Design review of the part built by this model. Coordinates are the model's own, in mm. Coordinates: 2 decimals unless noted, no trailing zeros. Write each loop counter-clockwise with the first axis right and the second up, starting at its lowest first coordinate (ties: lowest second). Pieces come first, ordered by that corner, then holes. Notation, with made-up numbers: (41.25, 32) -> (92.25, 32) arc R11 ccw to (92.25, 43) -> close; hole circle Ø6 at (-16.5, 19). An arc over 180 degrees is marked (long way). Answer in a Markdown table with one row per item. Add a question column.
Item 1: Take a section at A-A, the plane z = 59.5. Write out the cut boundary in (x, y) (3 decimals).
Item 2: Take a section at C-C, the plane x = 2.55. Give the number of separate pieces and of enclosed holes in the cut face, and give its area (3 significant figures).
Item 3: To check wall thickness, follow line 1 (Y direction, x = 2.7, z = -76); line 2 (Y direction, x = 1.95, z = 0); line 3 (Y direction, x = 0.8, z = 137.5). State the ranges of each line that lie inside material, in increasing order.
Item 4: Take a section at B-B, the plane y = 7.5. Write out the cut boundary in (x, z) (3 decimals), and give its area (3 significant figures).
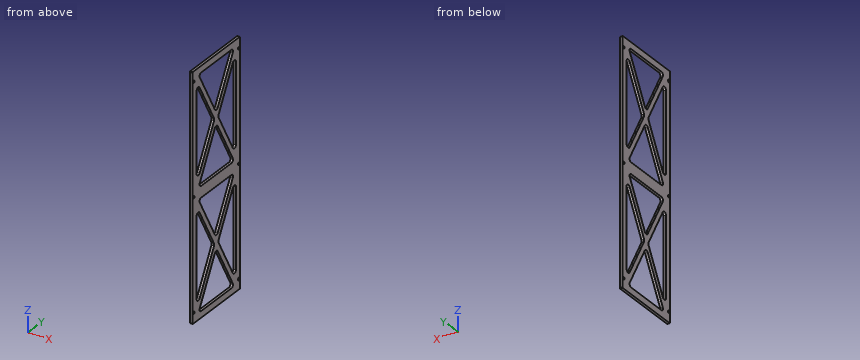
from build123d import *

# Parameters (mm, degrees)
SKETCH2_W            = 300
SKETCH2_H            = 90
BOSS_EXTRUDE1_DEPTH  = 3.175
CUT_EXTRUDE2_DEPTH   = 157.636779286
M3_CLEARANCE_HOLE1_D = 3.2
FILLET1_R            = 3
FILLET2_R            = 1


with BuildPart() as part:
    # Sketch2 → Boss-Extrude1 (new body)
    with BuildSketch(Plane(origin=(0, 0, 0), x_dir=(0, 0, -1), z_dir=(1, 0, 0))):
        Rectangle(SKETCH2_W, SKETCH2_H)
    extrude(amount=BOSS_EXTRUDE1_DEPTH)

    # Sketch4 → Cut-Extrude2 (cut, through all)
    with BuildSketch(Plane(origin=(3.175, 0, 0), x_dir=(0, 0, -1), z_dir=(1, 0, 0))):
        Polygon((-135.758731446, 37), (-13.241268554, 37), (-74.5, 3.4211398), align=None)
        Polygon((-7, 33.5788602), (-7, -33.5788602), (-68.258731446, 0), align=None)
        Polygon((-13.241268554, -37), (-135.758731446, -37), (-74.5, -3.4211398), align=None)
        Polygon((-142, -33.5788602), (-142, 33.5788602), (-80.741268554, 0), align=None)
        Polygon((135.758731446, 37), (13.241268554, 37), (74.5, 3.4211398), align=None)
        Polygon((142, 33.5788602), (80.741268554, 0), (142, -33.5788602), align=None)
        Polygon((135.758731446, -37), (74.5, -3.4211398), (13.241268554, -37), align=None)
        Polygon((7, -33.5788602), (68.258731446, 0), (7, 33.5788602), align=None)
    extrude(amount=-CUT_EXTRUDE2_DEPTH, mode=Mode.SUBTRACT)

    # M3 Clearance Hole1 (through all)
    with Locations(Plane(origin=(3.175, 0, 0), x_dir=(0, 0, -1), z_dir=(1, 0, 0))):
        with Locations((-137.5, 42.61875), (137.5, 42.61875), (137.5, -42.61875), (-137.5, -42.61875), (0, 42.61875), (0, -42.61875)):
            Hole(M3_CLEARANCE_HOLE1_D / 2)

    # Fillet1
    fillet1_edges = [part.edges().sort_by_distance(p)[0] for p in [
        (1.5875, 37, -135.758731446),
        (1.5875, 3.4211398, -74.5),
        (1.5875, 37, -13.241268554),
        (1.5875, 0, 80.741268554),
        (1.5875, -33.5788602, 142),
        (1.5875, 33.5788602, 142),
        (1.5875, 0, 68.258731446),
        (1.5875, 33.5788602, 7),
        (1.5875, -33.5788602, 7),
        (1.5875, -3.4211398, 74.5),
        (1.5875, -37, 13.241268554),
        (1.5875, -37, 135.758731446),
        (1.5875, -33.5788602, -7),
        (1.5875, 33.5788602, -7),
        (1.5875, 0, -68.258731446),
        (1.5875, 33.5788602, -142),
        (1.5875, -33.5788602, -142),
        (1.5875, 0, -80.741268554),
        (1.5875, -37, -135.758731446),
        (1.5875, -37, -13.241268554),
        (1.5875, -3.4211398, -74.5),
        (1.5875, 3.4211398, 74.5),
        (1.5875, 37, 135.758731446),
        (1.5875, 37, 13.241268554),
    ]]
    fillet(fillet1_edges, radius=FILLET1_R)

    # Fillet2
    fillet2_edges = [part.edges().sort_by_distance(p)[0] for p in [
        (1.5875, -45, -150),
        (1.5875, -45, 150),
        (1.5875, 45, 150),
        (1.5875, 45, -150),
    ]]
    fillet(fillet2_edges, radius=FILLET2_R)


solid = part.part
Answers:
| question | item | result |
|---|---|---|
| 1 | outline | (0, -45) -> (3.175, -45) -> (3.175, -37) -> (0, -37) -> close; (0, -11.643) -> (3.175, -11.643) -> (3.175, -4.801) -> (0, -4.801) -> close; (0, 4.801) -> (3.175, 4.801) -> (3.175, 11.643) -> (0, 11.643) -> close; (0, 37) -> (3.175, 37) -> (3.175, 45) -> (0, 45) -> close |
| 2 | separate pieces | 1 |
| 2 | enclosed holes | 14 |
| 2 | area | 10,800 mm^2 |
| 3 | line 1 | y = -45 to -37, -4.24 to 4.24, 37 to 45 |
| 3 | line 2 | y = -45 to -44.22, -41.02 to 41.02, 44.22 to 45 |
| 3 | line 3 | y = -45 to -44.22, -41.02 to -31.11, 31.11 to 41.02, 44.22 to 45 |
| 4 | outline | (0, -150) -> (3.175, -150) -> (3.175, -142) -> (0, -142) -> close; (0, -94.424) -> (3.175, -94.424) -> (3.175, -81.941) -> (0, -81.941) -> close; (0, -67.059) -> (3.175, -67.059) -> (3.175, -54.576) -> (0, -54.576) -> close; (0, -7) -> (3.175, -7) -> (3.175, 7) -> (0, 7) -> close; (0, 54.576) -> (3.175, 54.576) -> (3.175, 67.059) -> (0, 67.059) -> close; (0, 81.941) -> (3.175, 81.941) -> (3.175, 94.424) -> (0, 94.424) -> close; (0, 142) -> (3.175, 142) -> (3.175, 150) -> (0, 150) -> close |
| 4 | area | 254 mm^2 |
